```python
from build123d import *

# Parameters (mm, degrees)
SKIZZE1_W                       = 45
SKIZZE1_H                       = 85
AUFSATZ_LINEAR_AUSTRAGEN1_DEPTH = 2
SKIZZE6_R                       = 1.6
SCHNITT_LINEAR_AUSTRAGEN2_DEPTH = 2
SKIZZE7_W                       = 35
SKIZZE7_H                       = 1.5
SCHNITT_LINEAR_AUSTRAGEN3_DEPTH = 10
SKIZZE8_W                       = 29
SKIZZE8_H                       = 37.5
SCHNITT_LINEAR_AUSTRAGEN4_DEPTH = 10


with BuildPart() as part:
    # Skizze1 → Aufsatz-Linear austragen1 (new body)
    with BuildSketch(Plane.XY):
        with Locations((22.5, 42.5)):
            Rectangle(SKIZZE1_W, SKIZZE1_H)
    extrude(amount=AUFSATZ_LINEAR_AUSTRAGEN1_DEPTH)

    # Skizze6 → Schnitt-Linear austragen2 (cut)
    with BuildSketch(Plane.XY.offset(2)):
        with Locations((6, 80)):
            Circle(SKIZZE6_R)
        with Locations((39, 80)):
            Circle(SKIZZE6_R)
        with Locations((39, 5)):
            Circle(SKIZZE6_R)
        with Locations((6, 5)):
            Circle(SKIZZE6_R)
    extrude(amount=-SCHNITT_LINEAR_AUSTRAGEN2_DEPTH, mode=Mode.SUBTRACT)

    # Skizze7 → Schnitt-Linear austragen3 (cut)
    with BuildSketch(Plane.XY.offset(2)):
        with Locations((22.5, 58.8)):
            Rectangle(SKIZZE7_W, SKIZZE7_H)
        with Locations((22.5, 54.8)):
            Rectangle(SKIZZE7_W, SKIZZE7_H)
        with Locations((22.5, 50.8)):
            Rectangle(SKIZZE7_W, SKIZZE7_H)
        with Locations((22.5, 46.8)):
            Rectangle(SKIZZE7_W, SKIZZE7_H)
        with Locations((22.5, 42.8)):
            Rectangle(SKIZZE7_W, SKIZZE7_H)
        with Locations((22.5, 38.8)):
            Rectangle(SKIZZE7_W, SKIZZE7_H)
        with Locations((22.5, 34.8)):
            Rectangle(SKIZZE7_W, SKIZZE7_H)
        with Locations((22.5, 30.8)):
            Rectangle(SKIZZE7_W, SKIZZE7_H)
        with Locations((22.5, 26.8)):
            Rectangle(SKIZZE7_W, SKIZZE7_H)
        with Locations((22.5, 22.8)):
            Rectangle(SKIZZE7_W, SKIZZE7_H)
    extrude(amount=-SCHNITT_LINEAR_AUSTRAGEN3_DEPTH, mode=Mode.SUBTRACT)

    # Skizze8 → Schnitt-Linear austragen4 (cut)
    with BuildSketch(Plane.XY.offset(2)):
        with Locations((22.5, 40.8)):
            Rectangle(SKIZZE8_W, SKIZZE8_H)
    extrude(amount=-SCHNITT_LINEAR_AUSTRAGEN4_DEPTH, mode=Mode.SUBTRACT)


solid = part.part
```
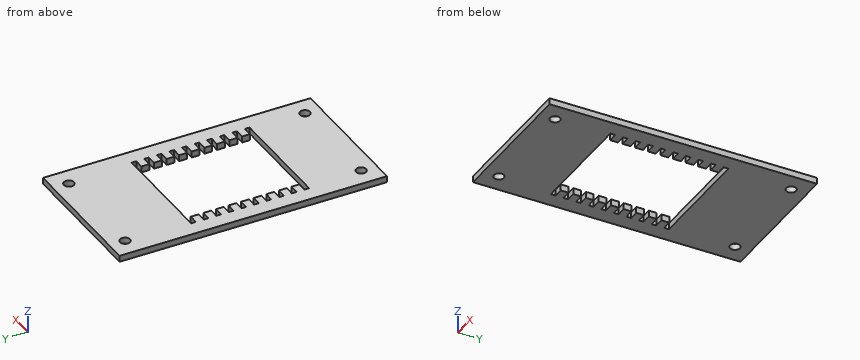
Can you work these out from the model? Positions are in its coordinate system, mm. Give positions to 0.01 mm unless a question says otherwise; leave off trailing zeros. Loops run counter-clockwise (first coordinate to the right, second up) from the corner with the lowest first, then second, coordinate; pieces in that order, holes last. Notation, with made-up numbers: M 50.5,-30.75 L 95.5,-30.75 A21 ccw 95.5,-11.75 Z; hole C 54,58.5 d5. An arc over 180 degrees is marked long. One line per question, with ' | ' between items. Start each with the question number.
Q1. If we section it at A-A (y = 5): Please give me the cut outline in (x, z), plus the area to 3 significant figures.
Q2. For pin 1 Ø2.5 at (x, y) = (6, 80) entering from +Z, with a flat end and sliding along its axis, tell me the tip position at first contact or that it passes through.
Q3. If I drill on line 1 (Y direction, x = 9, z = 1.3); line 2 (X direction, y = 28, z = 0.4); line 3 (X direction, y = 80, z = 1.4), over which ranges is the centre line in solid material (lowest first)? Write a range as from..to.
Q4. If we section it at D-D (x = 6): State how many separate pieces and enclosed holes the cut face has, plus the area to 3 significant figures.
Q5. If we section it at C-C (y = 37): Please give me the cut outline in (x, z), plus the area to 3 significant figures.
Q6. If we section it at B-B (x = 31.5): Please give me the cut outline in (y, z).
Computed:
1) outline: M 0,0 L 4.4,0 L 4.4,2 L 0,2 Z; M 7.6,0 L 37.4,0 L 37.4,2 L 7.6,2 Z; M 40.6,0 L 45,0 L 45,2 L 40.6,2 Z | area: 77.2 mm²
2) pin 1: passes through
3) line 1: y = 0..22.05, 59.55..85 | line 2: x = 0..8, 37..45 | line 3: x = 0..4.4, 7.6..37.4, 40.6..45
4) separate pieces: 13 | enclosed holes: 0 | area: 127 mm²
5) outline: M 0,0 L 8,0 L 8,2 L 0,2 Z; M 37,0 L 45,0 L 45,2 L 37,2 Z | area: 32.0 mm²
6) outline: M 0,0 L 22.05,0 L 22.05,2 L 0,2 Z; M 59.55,0 L 85,0 L 85,2 L 59.55,2 Z
